Part model, mm, in its own coordinate system. A direction names the side the tool comes from. Coordinates: 2 decimals unless noted, no trailing zeros. Write each loop counter-clockwise with the first axis right and the second up, starting at its lowest first coordinate (ties: lowest second). Pieces come first, ordered by that corner, then holes. Notation, with made-up numbers: (4.25, 75) -> (12.25, 75) arc R17 ccw to (12.25, 87) -> close; hole circle Ø1 at (-36.5, 61.5). An arc over 180 degrees is marked (long way). Write item = value, one per line.
from build123d import *

# Parameters (mm, degrees)
F0_R     = 6.35
F1_DEPTH = 19.05


with BuildPart() as f1:
    # F0 (on Top) → F1 (new body)
    with BuildSketch(Plane.XY):
        with BuildLine():
            ThreePointArc((61.064257, 17.418569), (62.535292, 11.026659), (63.339133, 4.517105))
            ThreePointArc((63.339133, 4.517105), (69.605701, 6.955225), (75.520491, 10.153593))
            ThreePointArc((75.520491, 10.153593), (75.042351, 13.231991), (74.438781, 16.288273))
            ThreePointArc((74.438781, 16.288273), (67.78679, 17.270778), (61.064257, 17.418569))
        make_face()
        with BuildLine():
            ThreePointArc((51.42413, 37.253307), (54.992613, 31.75), (57.974375, 25.90795))
            ThreePointArc((57.974375, 25.90795), (63.029136, 30.342325), (67.493315, 35.370785))
            ThreePointArc((67.493315, 35.370785), (65.991136, 38.1), (64.378656, 40.765533))
            ThreePointArc((64.378656, 40.765533), (57.791793, 39.413671), (51.42413, 37.253307))
        make_face()
        with BuildLine():
            ThreePointArc((35.581494, 52.594746), (40.817013, 48.643822), (45.617052, 44.173913))
            ThreePointArc((45.617052, 44.173913), (48.850328, 50.069693), (51.325449, 56.321739))
            ThreePointArc((51.325449, 56.321739), (48.980416, 58.372587), (46.553515, 60.325867))
            ThreePointArc((46.553515, 60.325867), (40.826252, 56.802693), (35.581494, 52.594746))
        make_face()
        with BuildLine():
            ThreePointArc((15.447205, 61.592482), (21.718279, 59.670481), (27.757639, 57.111851))
            ThreePointArc((27.757639, 57.111851), (28.779449, 63.757918), (28.966976, 70.47946))
            ThreePointArc((28.966976, 70.47946), (26.061935, 71.604578), (23.113332, 72.610012))
            ThreePointArc((23.113332, 72.610012), (18.936463, 67.340472), (15.447205, 61.592482))
        make_face()
        with BuildLine():
            ThreePointArc((-6.550245, 63.161256), (0, 63.5), (6.550245, 63.161256))
            ThreePointArc((6.550245, 63.161256), (5.237344, 69.755996), (3.114659, 76.136318))
            ThreePointArc((3.114659, 76.136318), (0, 76.2), (-3.114659, 76.136318))
            ThreePointArc((-3.114659, 76.136318), (-5.237344, 69.755996), (-6.550245, 63.161256))
        make_face()
        with BuildLine():
            ThreePointArc((-27.757639, 57.111851), (-21.718279, 59.670481), (-15.447205, 61.592482))
            ThreePointArc((-15.447205, 61.592482), (-18.936463, 67.340472), (-23.113332, 72.610012))
            ThreePointArc((-23.113332, 72.610012), (-26.061935, 71.604578), (-28.966976, 70.47946))
            ThreePointArc((-28.966976, 70.47946), (-28.779449, 63.757918), (-27.757639, 57.111851))
        make_face()
        with BuildLine():
            ThreePointArc((-45.617052, 44.173913), (-40.817013, 48.643822), (-35.581494, 52.594746))
            ThreePointArc((-35.581494, 52.594746), (-40.826252, 56.802693), (-46.553515, 60.325867))
            ThreePointArc((-46.553515, 60.325867), (-48.980416, 58.372587), (-51.325449, 56.321739))
            ThreePointArc((-51.325449, 56.321739), (-48.850328, 50.069693), (-45.617052, 44.173913))
        make_face()
        with BuildLine():
            ThreePointArc((-57.974375, 25.90795), (-54.992613, 31.75), (-51.42413, 37.253307))
            ThreePointArc((-51.42413, 37.253307), (-57.791793, 39.413671), (-64.378656, 40.765533))
            ThreePointArc((-64.378656, 40.765533), (-65.991136, 38.1), (-67.493315, 35.370785))
            ThreePointArc((-67.493315, 35.370785), (-63.029136, 30.342325), (-57.974375, 25.90795))
        make_face()
        with BuildLine():
            ThreePointArc((-63.339133, 4.517105), (-62.535292, 11.026659), (-61.064257, 17.418569))
            ThreePointArc((-61.064257, 17.418569), (-67.78679, 17.270778), (-74.438781, 16.288273))
            ThreePointArc((-74.438781, 16.288273), (-75.042351, 13.231991), (-75.520491, 10.153593))
            ThreePointArc((-75.520491, 10.153593), (-69.605701, 6.955225), (-63.339133, 4.517105))
        make_face()
        with BuildLine():
            ThreePointArc((-74.438781, -16.288273), (-67.78679, -17.270778), (-61.064257, -17.418569))
            ThreePointArc((-61.064257, -17.418569), (-62.535292, -11.026659), (-63.339133, -4.517105))
            ThreePointArc((-63.339133, -4.517105), (-69.605701, -6.955225), (-75.520491, -10.153593))
            ThreePointArc((-75.520491, -10.153593), (-75.042351, -13.231991), (-74.438781, -16.288273))
        make_face()
        with BuildLine():
            ThreePointArc((-64.378656, -40.765533), (-57.791793, -39.413671), (-51.42413, -37.253307))
            ThreePointArc((-51.42413, -37.253307), (-54.992613, -31.75), (-57.974375, -25.90795))
            ThreePointArc((-57.974375, -25.90795), (-63.029136, -30.342325), (-67.493315, -35.370785))
            ThreePointArc((-67.493315, -35.370785), (-65.991136, -38.1), (-64.378656, -40.765533))
        make_face()
        with BuildLine():
            ThreePointArc((-46.553515, -60.325867), (-40.826252, -56.802693), (-35.581494, -52.594746))
            ThreePointArc((-35.581494, -52.594746), (-40.817013, -48.643822), (-45.617052, -44.173913))
            ThreePointArc((-45.617052, -44.173913), (-48.850328, -50.069693), (-51.325449, -56.321739))
            ThreePointArc((-51.325449, -56.321739), (-48.980416, -58.372587), (-46.553515, -60.325867))
        make_face()
        with BuildLine():
            ThreePointArc((-23.113332, -72.610012), (-18.936463, -67.340472), (-15.447205, -61.592482))
            ThreePointArc((-15.447205, -61.592482), (-21.718279, -59.670481), (-27.757639, -57.111851))
            ThreePointArc((-27.757639, -57.111851), (-28.779449, -63.757918), (-28.966976, -70.47946))
            ThreePointArc((-28.966976, -70.47946), (-26.061935, -71.604578), (-23.113332, -72.610012))
        make_face()
        with BuildLine():
            ThreePointArc((3.114659, -76.136318), (5.237344, -69.755996), (6.550245, -63.161256))
            ThreePointArc((6.550245, -63.161256), (0, -63.5), (-6.550245, -63.161256))
            ThreePointArc((-6.550245, -63.161256), (-5.237344, -69.755996), (-3.114659, -76.136318))
            ThreePointArc((-3.114659, -76.136318), (0, -76.2), (3.114659, -76.136318))
        make_face()
        with BuildLine():
            ThreePointArc((28.966976, -70.47946), (28.779449, -63.757918), (27.757639, -57.111851))
            ThreePointArc((27.757639, -57.111851), (21.718279, -59.670481), (15.447205, -61.592482))
            ThreePointArc((15.447205, -61.592482), (18.936463, -67.340472), (23.113332, -72.610012))
            ThreePointArc((23.113332, -72.610012), (26.061935, -71.604578), (28.966976, -70.47946))
        make_face()
        with BuildLine():
            ThreePointArc((51.325449, -56.321739), (48.850328, -50.069693), (45.617052, -44.173913))
            ThreePointArc((45.617052, -44.173913), (40.817013, -48.643822), (35.581494, -52.594746))
            ThreePointArc((35.581494, -52.594746), (40.826252, -56.802693), (46.553515, -60.325867))
            ThreePointArc((46.553515, -60.325867), (48.980416, -58.372587), (51.325449, -56.321739))
        make_face()
        with BuildLine():
            ThreePointArc((67.493315, -35.370785), (63.029136, -30.342325), (57.974375, -25.90795))
            ThreePointArc((57.974375, -25.90795), (54.992613, -31.75), (51.42413, -37.253307))
            ThreePointArc((51.42413, -37.253307), (57.791793, -39.413671), (64.378656, -40.765533))
            ThreePointArc((64.378656, -40.765533), (65.991136, -38.1), (67.493315, -35.370785))
        make_face()
        with BuildLine():
            ThreePointArc((75.520491, -10.153593), (69.605701, -6.955225), (63.339133, -4.517105))
            ThreePointArc((63.339133, -4.517105), (62.535292, -11.026659), (61.064257, -17.418569))
            ThreePointArc((61.064257, -17.418569), (67.78679, -17.270778), (74.438781, -16.288273))
            ThreePointArc((74.438781, -16.288273), (75.042351, -13.231991), (75.520491, -10.153593))
        make_face()
        with BuildLine():
            ThreePointArc((63.339133, -4.517105), (63.45977, -2.259984), (63.5, 0))
            ThreePointArc((63.5, 0), (63.45977, 2.259984), (63.339133, 4.517105))
            ThreePointArc((63.339133, 4.517105), (62.535292, 11.026659), (61.064257, 17.418569))
            ThreePointArc((61.064257, 17.418569), (59.670481, 21.718279), (57.974375, 25.90795))
            ThreePointArc((57.974375, 25.90795), (54.992613, 31.75), (51.42413, 37.253307))
            ThreePointArc((51.42413, 37.253307), (48.643822, 40.817013), (45.617052, 44.173913))
            ThreePointArc((45.617052, 44.173913), (40.817013, 48.643822), (35.581494, 52.594746))
            ThreePointArc((35.581494, 52.594746), (31.75, 54.992613), (27.757639, 57.111851))
            ThreePointArc((27.757639, 57.111851), (21.718279, 59.670481), (15.447205, 61.592482))
            ThreePointArc((15.447205, 61.592482), (11.026659, 62.535292), (6.550245, 63.161256))
            ThreePointArc((6.550245, 63.161256), (0, 63.5), (-6.550245, 63.161256))
            ThreePointArc((-6.550245, 63.161256), (-11.026659, 62.535292), (-15.447205, 61.592482))
            ThreePointArc((-15.447205, 61.592482), (-21.718279, 59.670481), (-27.757639, 57.111851))
            ThreePointArc((-27.757639, 57.111851), (-31.75, 54.992613), (-35.581494, 52.594746))
            ThreePointArc((-35.581494, 52.594746), (-40.817013, 48.643822), (-45.617052, 44.173913))
            ThreePointArc((-45.617052, 44.173913), (-48.643822, 40.817013), (-51.42413, 37.253307))
            ThreePointArc((-51.42413, 37.253307), (-54.992613, 31.75), (-57.974375, 25.90795))
            ThreePointArc((-57.974375, 25.90795), (-59.670481, 21.718279), (-61.064257, 17.418569))
            ThreePointArc((-61.064257, 17.418569), (-62.535292, 11.026659), (-63.339133, 4.517105))
            ThreePointArc((-63.339133, 4.517105), (-63.5, 0), (-63.339133, -4.517105))
            ThreePointArc((-63.339133, -4.517105), (-62.535292, -11.026659), (-61.064257, -17.418569))
            ThreePointArc((-61.064257, -17.418569), (-59.670481, -21.718279), (-57.974375, -25.90795))
            ThreePointArc((-57.974375, -25.90795), (-54.992613, -31.75), (-51.42413, -37.253307))
            ThreePointArc((-51.42413, -37.253307), (-48.643822, -40.817013), (-45.617052, -44.173913))
            ThreePointArc((-45.617052, -44.173913), (-40.817013, -48.643822), (-35.581494, -52.594746))
            ThreePointArc((-35.581494, -52.594746), (-31.75, -54.992613), (-27.757639, -57.111851))
            ThreePointArc((-27.757639, -57.111851), (-21.718279, -59.670481), (-15.447205, -61.592482))
            ThreePointArc((-15.447205, -61.592482), (-11.026659, -62.535292), (-6.550245, -63.161256))
            ThreePointArc((-6.550245, -63.161256), (0, -63.5), (6.550245, -63.161256))
            ThreePointArc((6.550245, -63.161256), (11.026659, -62.535292), (15.447205, -61.592482))
            ThreePointArc((15.447205, -61.592482), (21.718279, -59.670481), (27.757639, -57.111851))
            ThreePointArc((27.757639, -57.111851), (31.75, -54.992613), (35.581494, -52.594746))
            ThreePointArc((35.581494, -52.594746), (40.817013, -48.643822), (45.617052, -44.173913))
            ThreePointArc((45.617052, -44.173913), (48.643822, -40.817013), (51.42413, -37.253307))
            ThreePointArc((51.42413, -37.253307), (54.992613, -31.75), (57.974375, -25.90795))
            ThreePointArc((57.974375, -25.90795), (59.670481, -21.718279), (61.064257, -17.418569))
            ThreePointArc((61.064257, -17.418569), (62.535292, -11.026659), (63.339133, -4.517105))
        make_face()
        Circle(F0_R, mode=Mode.SUBTRACT)
    extrude(amount=F1_DEPTH)


solid = f1.part
Q1. Pin check, flat tips, straight feed: pin 1 (1.5 mm diameter, centred on y = -24.5, z = 13.5, fed in from -X); pin 2 (6 mm diameter, centred on x = -13, z = 13.5, fed in from -Y); pin 3 (6 mm diameter, centred on y = 24, z = 7.5, fed in from +X). Stop position of each tip, or through.
Model answer:
pin_1 = -58.89
pin_2 = -62.71
pin_3 = 59.93
Q2. Saw through at A-A on x = 0. Give the cut face in (y, z), and give its area (3 significant figures).
Model answer:
outline = (-76.2, 0) -> (-6.35, 0) -> (-6.35, 19.05) -> (-76.2, 19.05) -> close; (6.35, 0) -> (76.2, 0) -> (76.2, 19.05) -> (6.35, 19.05) -> close
area = 2,660 mm²
Q3. Probe line 1 (Y direction, x = 0, z = 8.5); line 2 (X direction, y = -58, z = 2.75); line 3 (Y direction, x = -2.5, z = 3.5). List the from-to ranges inside material, lowest first. Write a range as from..to.
Model answer:
line_1 = -76.2..-6.35, 6.35..76.2
line_2 = -49.42..-42.6, -27.94..27.94, 42.6..49.42
line_3 = -76.16..-5.84, 5.84..76.16
Q4. Which spindle directions (+Z, -Z, +X, -X, +Y, -Y) get a long thin tool onto all of the face, cutting with end or side? Do faces 4 (the face through (28.788, -63.852, 9.392)), 5 (the face through (-18.99, -67.42, 9.39)), 6 (the face through (11.089, 62.524, 9.392)), 7 (the face through (48.81, 49.98, 9.39)). Say none if no direction does.
Model answer:
face_4 = +Z, -Z
face_5 = +Z, -Z, -Y
face_6 = +Z, -Z, +Y
face_7 = +Z, -Z, +X
Q5. Mould opens along X. For faces 1 (the face through (-48.95, 58.4, 9.39)), 2 (the face through (59.65, -21.78, 9.39)), 3 (the face through (-10.964, 62.546, 9.392)) say: released by +X, released by -X, zero draft, split by the parting line, or undercut.
Model answer:
face_1 = released by -X
face_2 = released by +X
face_3 = undercut
